The model under review builds one solid part; all positions refer to its coordinate system, in mm. Face numbers are marked on the shaded views. A direction names the side the tool comes from. Coordinates: 2 decimals unless noted, no trailing zeros. Write each loop counter-clockwise with the first axis right and the second up, starting at its lowest first coordinate (ties: lowest second). Pieces come first, ordered by that corner, then holes. Notation, with made-up numbers: (17, -26) - (65, -26) arc R19 cw to (65, 6) - close; hole circle Ø10 at (73.5, 44). An arc over 180 degrees is marked (long way). Return JSON: item names as keys, results as strings. Group by question number.
(1) Tool access review of the marked faces 1, 2 and 3: name each direction out of +Z, -Z, +X, -X, +Y, -Y from which nothing blocks a thin tool from reaching the whole face with its end or side.
(2) For pin 1 Ø6 at (y, z) = (-6, 9) entering from +X; pin 2 Ø3 at (x, z) = (6, 4.5) entering from -Y; pin 3 Ø3.5 at (x, z) = (3, 9) entering from +Y, all flat-tipped, find the tip position at first contact; note any pin that passes through.
(3) To check wall thickness, follow L1, parallel to X at y = 7.5, z = 4; L2, parallel to Y at x = 0, z = 8.05; L3, parallel to X at y = 0, z = 7.3. State the ranges of each line that lie inside material, in increasing order. Write a range as from..to.
(4) Draft analysis for pull direction X (two halves, no side actions). For the marked faces 4, 5, 6 and 7, state which applies: released by +X, released by -X, zero draft, split by the parting line, or undercut.
(5) We need section A-A on x = 0. State the section outline as (y, z) points.
(6) We need section B-B on y = 0. State the section outline as (x, z) points.
(7) We need section D-D on x = -4.5. State the section outline as (y, z) points, then the cut area to 3 significant figures.
(8) We need section C-C on z = 8.25. State the section outline as (x, y) points.
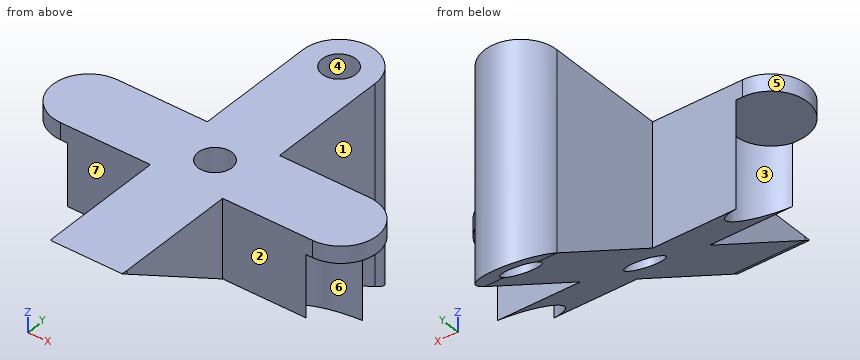
```python
from build123d import *

# Parameters (mm, degrees)
F0_W          = 4.28
F0_H          = 3.44
F0_W_2        = 3.44
F0_H_2        = 5.78
F1_DEPTH      = 12
F3_DEPTH      = 25
F3_DEPTH_BACK = 25
F5_R          = 0.8
F6_DEPTH      = 55
F7_W          = 30.6417569518
F7_H          = 23.9444840699
F8_DEPTH      = 1.5
F9_R          = 0.8
F10_DEPTH     = 10.501
F4_R          = 1.75
F12_DEPTH     = 9.7


with BuildPart() as f1:
    # F0 (on Top) → F1 (new body)
    with BuildSketch(Plane.XY):
        with Locations((3.86, 0)):
            Rectangle(F0_W, F0_H)
        with BuildLine():
            Line((6, 1.72), (6, -1.72))
            ThreePointArc((6, -1.72), (7.72, 0), (6, 1.72))
        make_face()
        with Locations((0, -4.61)):
            Rectangle(F0_W_2, F0_H_2)
        Rectangle(F0_W_2, F0_H)
        with Locations((-3.86, 0)):
            Rectangle(F0_W, F0_H)
        with BuildLine():
            ThreePointArc((-1.72, -7.5), (0, -9.22), (1.72, -7.5))
            Line((1.72, -7.5), (-1.72, -7.5))
        make_face()
        with Locations((0, 4.61)):
            Rectangle(F0_W_2, F0_H_2)
        with BuildLine():
            ThreePointArc((-6, 1.72), (-7.72, 0), (-6, -1.72))
            Line((-6, -1.72), (-6, 1.72))
        make_face()
        with BuildLine():
            Line((-1.72, 7.5), (1.72, 7.5))
            ThreePointArc((1.72, 7.5), (0, 9.22), (-1.72, 7.5))
        make_face()
    extrude(amount=F1_DEPTH)

    # F2 (on Right) → F3 (cut, two sides)
    with BuildSketch(Plane.YZ) as f3_sk:
        Polygon((-7.5, 0), (7.5, 0), (7.5, 1.0621960754), (-7.5, 10.3255339419), align=None)
        Polygon((7.5, 1.0621960754), (7.5, 0), (9.22, 0), align=None)
        Polygon((-9.22, 0), (-7.5, 0), (-7.5, 10.3255339419), (-9.22, 11.3877300173), align=None)
    extrude(amount=-F3_DEPTH, mode=Mode.SUBTRACT)
    extrude(f3_sk.sketch, amount=F3_DEPTH_BACK, mode=Mode.SUBTRACT)

    # F5 (on Top) → F6 (cut)
    with BuildSketch(Plane.XY):
        Circle(F5_R)
    extrude(amount=F6_DEPTH, mode=Mode.SUBTRACT)

    # F7 (on face) → F8 (cut)
    with BuildSketch(Plane.XY.offset(12)):
        Rectangle(F7_W, F7_H)
    extrude(amount=-F8_DEPTH, mode=Mode.SUBTRACT)

    # F9 (on face) → F10 (cut, through all)
    with BuildSketch(Plane.XY.offset(10.5)):
        with Locations((0, 7.5)):
            Circle(F9_R)
    extrude(amount=-F10_DEPTH, mode=Mode.SUBTRACT)

    # F4 (on Top) → F12 (cut)
    with BuildSketch(Plane.XY):
        with Locations((6, 0)):
            Circle(F4_R)
        with Locations((-6, 0)):
            Circle(F4_R)
    extrude(amount=F12_DEPTH, mode=Mode.SUBTRACT)


solid = f1.part
```
Ans:
{
 "1": {"face 1": "+Z, -Z, +X, +Y", "face 2": "+Z, -Z, +X, -Y", "face 3": "-Z, -X"},
 "2": {"pin 1": "x = 1.72", "pin 2": "y = 1.05", "pin 3": "y = 8.68"},
 "3": {"L1": "-1.72..-0.8, 0.8..1.72", "L2": "-3.82..-0.8, 0.8..6.7, 8.3..9.22", "L3": "-4.25..-0.8, 0.8..4.25"},
 "4": {"face 4": "undercut", "face 5": "released by -X", "face 6": "released by +X", "face 7": "zero draft"},
 "5": {"outline": "(-7.78, 10.5) - (-0.8, 6.19) - (-0.8, 10.5) - close; (0.8, 5.2) - (6.7, 1.56) - (6.7, 10.5) - (0.8, 10.5) - close; (8.3, 0.57) - (9.22, 0) - (9.22, 10.5) - (8.3, 10.5) - close"},
 "6": {"outline": "(-7.72, 9.7) - (-4.25, 9.7) - (-4.25, 5.69) - (-0.8, 5.69) - (-0.8, 10.5) - (-7.72, 10.5) - close; (0.8, 5.69) - (4.25, 5.69) - (4.25, 9.7) - (7.72, 9.7) - (7.72, 10.5) - (0.8, 10.5) - close"},
 "7": {"outline": "(-1.72, 6.76) - (-0.9, 6.25) - (-0.9, 9.7) - (0.9, 9.7) - (0.9, 5.14) - (1.72, 4.63) - (1.72, 10.5) - (-1.72, 10.5) - close", "area": "9.31 mm²"},
 "8": {"outline": "(-5.68, -1.72) - (-1.72, -1.72) - (-1.72, -4.14) - (1.72, -4.14) - (1.72, -1.72) - (5.68, -1.72) arc R1.75 cw to (5.68, 1.72) - (1.72, 1.72) - (1.72, 7.5) arc R1.72 ccw to (-1.72, 7.5) - (-1.72, 1.72) - (-5.68, 1.72) arc R1.75 cw to start; hole circle Ø1.6 at (0, 0); hole circle Ø1.6 at (0, 7.5)"}
}
